from build123d import *

# Parameters (mm, degrees)
BOSS_EXTRUDE11_DEPTH = 12.7
BOSS_EXTRUDE12_DEPTH = 12.7
BOSS_EXTRUDE13_DEPTH = 12.7
CUT_EXTRUDE1_START   = 12.7
CUT_EXTRUDE1_DEPTH   = 6.858
SKETCH25_R           = 1.90000001
CUT_EXTRUDE2_DEPTH   = 13.7
FILLET1_R            = 2.54
FILLET2_R            = 6.35


with BuildPart() as part:
    # Sketch12 → Boss-Extrude11 (new body)
    with BuildSketch(Plane(origin=(0, 0, 0), x_dir=(1, 0, 0), z_dir=(0, 1, 0))):
        Polygon((139.879605122, 6.35), (6.529605122, 6.35), (0.179605122, 0), (6.529605122, -6.35), (139.879605122, -6.35), align=None)
    extrude(amount=BOSS_EXTRUDE11_DEPTH)

    # Sketch23 → Boss-Extrude12 (add)
    with BuildSketch(Plane(origin=(0, 0, 0), x_dir=(1, 0, 0), z_dir=(0, 1, 0))):
        Polygon((90.5209817, 0), (124.090746971, 33.569765271), (157.660512242, 0), (124.090746971, -33.569765271), align=None)
    extrude(amount=BOSS_EXTRUDE12_DEPTH)

    # Sketch26 → Boss-Extrude13 (add)
    with BuildSketch(Plane(origin=(0, 0, 0), x_dir=(1, 0, 0), z_dir=(0, 1, 0))):
        with BuildLine():
            Line((22.540263258, 22.360658136), (0.179605122, 0))
            Line((0.179605122, 0), (22.540263258, -22.360658136))
            ThreePointArc((22.540263258, -22.360658136), (31.75, 0), (22.540263258, 22.360658136))
        make_face()
    extrude(amount=BOSS_EXTRUDE13_DEPTH)

    # Sketch24 → Cut-Extrude1 (cut)
    with BuildSketch(Plane(origin=(0, 0, 0), x_dir=(1, 0, 0), z_dir=(0, 1, 0)).offset(CUT_EXTRUDE1_START)):
        Polygon((119.780224033, 29.259242333), (149.039466366, 0), (119.780224033, -29.259242333), (110.440757667, -19.919775967), (130.360533634, 0), (110.440757667, 19.919775967), align=None)
    extrude(amount=-CUT_EXTRUDE1_DEPTH, mode=Mode.SUBTRACT)

    # Sketch25 → Cut-Extrude2 (cut, through all)
    with BuildSketch(Plane(origin=(0, 0, 0), x_dir=(1, 0, 0), z_dir=(0, 1, 0))):
        with Locations((21.997045256, 12.7)):
            Circle(SKETCH25_R)
        with Locations((21.997045256, -12.7)):
            Circle(SKETCH25_R)
    extrude(amount=CUT_EXTRUDE2_DEPTH, mode=Mode.SUBTRACT)

    # Fillet1
    fillet1_edges = [part.edges().sort_by_distance(p)[0] for p in [
        (120.400645651, 12.7, 9.959887983),
        (120.400645651, 12.7, -9.959887983),
        (134.4098452, 12.7, -14.629621166),
        (134.4098452, 12.7, 14.629621166),
    ]]
    fillet(fillet1_edges, radius=FILLET1_R)

    # Fillet2
    fillet2_edges = [part.edges().sort_by_distance(p)[0] for p in [
        (96.8709817, 6.35, 6.35),
        (96.8709817, 6.35, -6.35),
        (31.108519733, 6.35, -6.35),
        (31.108519733, 6.35, 6.35),
    ]]
    fillet(fillet2_edges, radius=FILLET2_R)


solid = part.part
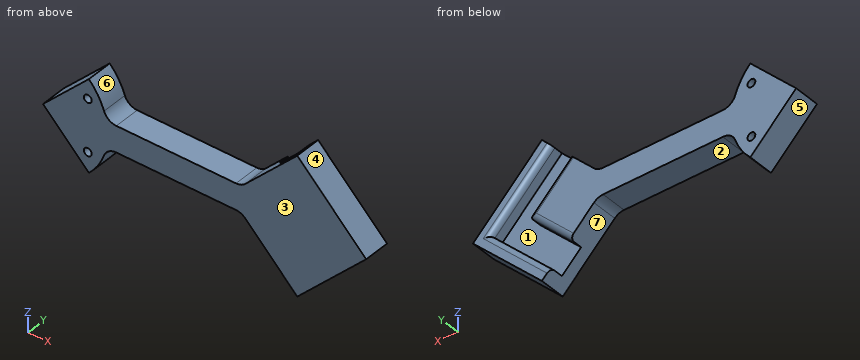
Design review of the part built by this model. Coordinates are the model's own, in mm. Face numbers are marked on the shaded views. A direction names the side the tool comes from. Give positions to 0.01 mm unless a question says otherwise; leave off trailing zeros. Loops run counter-clockwise (first coordinate to the right, second up) from the corner with the lowest first, then second, coordinate; pieces in that order, holes last. Notation, with made-up numbers: M 83.5,-18 L 91.5,-18 A8 cw 91.5,-13 Z; hole C 45.5,36.25 d7. An arc over 180 degrees is marked long. Answer as a JSON object with one key per item and string values.
Item 1: We need section D-D (x = 48). State the section outline as (y, z) points, and give its area (3 significant figures).
Output values:
{"outline": "M 0,-6.35 L 12.7,-6.35 L 12.7,6.35 L 0,6.35 Z", "area": "161 mm2"}
Item 2: We need section A-A (y = 8.5). State the section outline as (x, z) points, and give its area (3 significant figures).
Output values:
{"outline": "M 0.18,0 L 22.54,-22.36 A31.75 ccw 29.93,-10.58 A6.35 cw 35.92,-6.35 L 94.24,-6.35 A6.35 cw 98.73,-8.21 L 110.44,-19.92 L 130.36,0 L 110.44,19.92 L 98.73,8.21 A6.35 cw 94.24,6.35 L 35.92,6.35 A6.35 cw 29.93,10.58 A31.75 ccw 22.54,22.36 Z; M 119.78,-29.26 L 124.09,-33.57 L 157.66,0 L 124.09,33.57 L 119.78,29.26 L 149.04,0 Z; hole C 22,-12.7 d3.8; hole C 22,12.7 d3.8", "area": "2,900 mm2"}
Item 3: We need section C-C (z = 12.7). Count the separate pieces of the cut face and the enclosed holes in it, and give its area (3 significant figures).
Output values:
{"separate pieces": "3", "enclosed holes": "0", "area": "556 mm2"}
Item 4: Mouldability with a two-part tool opening along Z and no side actions: class the marked faces 1, 2, 3 and 4 as pulls with the +Z half, pulls with the -Z half, needs draft (parallel to the pull), parting line crosses it, or undercut.
Output values:
{"face 1": "undercut", "face 2": "pulls with the -Z half", "face 3": "needs draft", "face 4": "pulls with the +Z half"}
Item 5: For P1, Ø1.5, axis at y = 7.5, z = -25, coming from the -X side; P2, Ø4, axis at y = 11, z = -25, coming from the +X side; P3, Ø4, axis at x = 64.5, y = 7.5, coming from the +Z side, all flat-tipped, find the tip position at first contact; note any pin that passes through.
Output values:
{"P1": "stops at x = 123.29", "P2": "stops at x = 134.66", "P3": "stops at z = 6.35"}
Item 6: We need section B-B (y = 1.75). State the section outline as (x, z) points, and give its area (3 significant figures).
Output values:
{"outline": "M 0.18,0 L 22.54,-22.36 A31.75 ccw 29.93,-10.58 A6.35 cw 35.92,-6.35 L 94.24,-6.35 A6.35 cw 98.73,-8.21 L 124.09,-33.57 L 157.66,0 L 124.09,33.57 L 98.73,8.21 A6.35 cw 94.24,6.35 L 35.92,6.35 A6.35 cw 29.93,10.58 A31.75 ccw 22.54,22.36 Z; hole C 22,-12.7 d3.8; hole C 22,12.7 d3.8", "area": "3,810 mm2"}
Item 7: Wall thickness on line 1 along X through (y, z) = (6.25, -12.7); line 2 along X through (y, z) = (5.5, 12.7); line 3 along Z through (x, y) = (120.5, 6.5): over which ranges is each line inside the solid? List them lowest first.
Output values:
{"line 1": "x = 12.88 to 20.1, 23.9 to 29.1, 103.22 to 117.66, 136.34 to 144.96", "line 2": "x = 12.88 to 20.1, 23.9 to 29.1, 103.22 to 144.96", "line 3": "z = -29.98 to -28.54, -9.86 to 9.86, 28.54 to 29.98"}
Item 8: Machinability: for the marked faces 5, 6 and 7, which of the approach directions +Z, -Z, +X, -X, +Y, -Y give a long, thin tool a straight path to every point of the face, cutting with its end or side? Answer none if there is none.
Output values:
{"face 5": "-Z, -X, +Y, -Y", "face 6": "+Z, +Y, -Y", "face 7": "-Z, +Y, -Y"}
